Verification items for the finished model (mm, model axes). A direction names the side the tool comes from. Coordinates: 2 decimals unless noted, no trailing zeros. Write each loop counter-clockwise with the first axis right and the second up, starting at its lowest first coordinate (ties: lowest second). Pieces come first, ordered by that corner, then holes. Notation, with made-up numbers: (45, -33) -> (55, -33) arc R11 cw to (55, -26) -> close; hole circle Ø5 at (58.25, 29.25). An arc over 180 degrees is marked (long way). Write item = value, one per line. Start each with the question number.
(1) Section check B-B (y = 37.5). Record the cut outline in (x, z).
(2) Section check A-A (z = 63). Record the cut outline in (x, y).
(3) Section check C-C (x = 697). Record the cut outline in (y, z).
(4) Mould release check, pull along Y, two halves, no side actions. Record for faces 1 (the face through (766.989, 46, 42)), 2 (the face through (760.948, 70.986, 39.97)), 3 (the face through (773.5, 52.48, 35.85)): released by +Y, released by -Y, zero draft, split by the parting line, or undercut.
(5) Set-up check for faces 4 (the face through (757.88, 30.04, 44.06)), 5 (the face through (774.927, 57, 38)): record each of +Z, -Z, +X, -X, +Y, -Y from which the full face is reachable in a straight line by a thin tool's end or side.
(6) Material ranges on probe 1 along X at (y, z) = (77.5, 21); probe 2 along Y at (x, z) = (764, 38.5); probe 3 along Y at (x, z) = (758.5, 19), recorded low to high. Write a range as [from, to].
(7) Gauge pin test, flat ends, axial feed: pin 1 Ø10 at (y, z) = (47, 49) entering from +X; pin 2 Ø8 at (x, y) = (684.5, 50) entering from -Z; pin 3 Ø11.5 at (y, z) = (62.5, 42) entering from +X; pin 4 Ø5 at (x, y) = (759.5, 71.5) entering from -Z. Record the tip position at first contact, or that the pin passes through.
```python
from build123d import *


with BuildPart() as part:
    # Sketch1 → Revolve1 (revolve)
    with BuildSketch(Plane.XY.offset(38.109948098), mode=Mode.PRIVATE) as revolve1_sk:
        with BuildLine():
            Line((670.54800115, 86.792545046), (670.54800115, 56.820545046))
            Line((670.54800115, 56.820545046), (774.926761151, 56.820545046))
            Line((774.926761151, 56.820545046), (774.926761151, 59.38835011))
            ThreePointArc((774.926761151, 59.38835011), (774.645765826, 60.549598522), (773.8649518, 61.453913569))
            Line((773.8649518, 61.453913569), (768.0510705, 65.614533734))
            ThreePointArc((768.0510705, 65.614533734), (767.270256474, 66.518848781), (766.98926115, 67.680097193))
            Line((766.98926115, 67.680097193), (766.98926115, 68.568045046))
            ThreePointArc((766.98926115, 68.568045046), (766.245312374, 70.36409627), (764.44926115, 71.108045046))
            Line((764.44926115, 71.108045046), (757.54300115, 71.108045046))
            ThreePointArc((757.54300115, 71.108045046), (756.644975538, 71.480019434), (756.27300115, 72.378045046))
            Line((756.27300115, 72.378045046), (756.27300115, 84.252545046))
            Line((756.27300115, 84.252545046), (759.44800115, 84.252545046))
            Line((759.44800115, 84.252545046), (759.44800115, 86.792545046))
            Line((759.44800115, 86.792545046), (670.54800115, 86.792545046))
        make_face()
    revolve(revolve1_sk.sketch.rotate(Axis((670.54800115, 56.820545046, 38.109948098), (1, 0, 0)), 270), axis=Axis((670.54800115, 56.820545046, 38.109948098), (1, 0, 0)))


solid = part.part
```
Response:
q1.outline = (670.55, 15.2) -> (759.45, 15.2) -> (759.45, 18.64) -> (756.27, 18.64) -> (756.27, 57.58) -> (759.45, 57.58) -> (759.45, 61.02) -> (670.55, 61.02) -> close
q2.outline = (670.55, 40.12) -> (759.45, 40.12) -> (759.45, 45.29) -> (756.27, 45.29) -> (756.27, 68.35) -> (759.45, 68.35) -> (759.45, 73.52) -> (670.55, 73.52) -> close
q3.outline = circle Ø59.94 at (56.82, 38.11)
q4.face_1 = zero draft
q4.face_2 = undercut
q4.face_3 = split by the parting line
q5.face_4 = +X
q5.face_5 = +Z, -Z, +X, +Y, -Y
q6.probe_1 = [670.55, 756.27]
q6.probe_2 = [42.54, 71.1]
q6.probe_3 = [33.73, 37.14], [76.5, 79.91]
q7.pin_1 = 767.29
q7.pin_2 = 8.27
q7.pin_3 = 774.93
q7.pin_4 = 10.72
